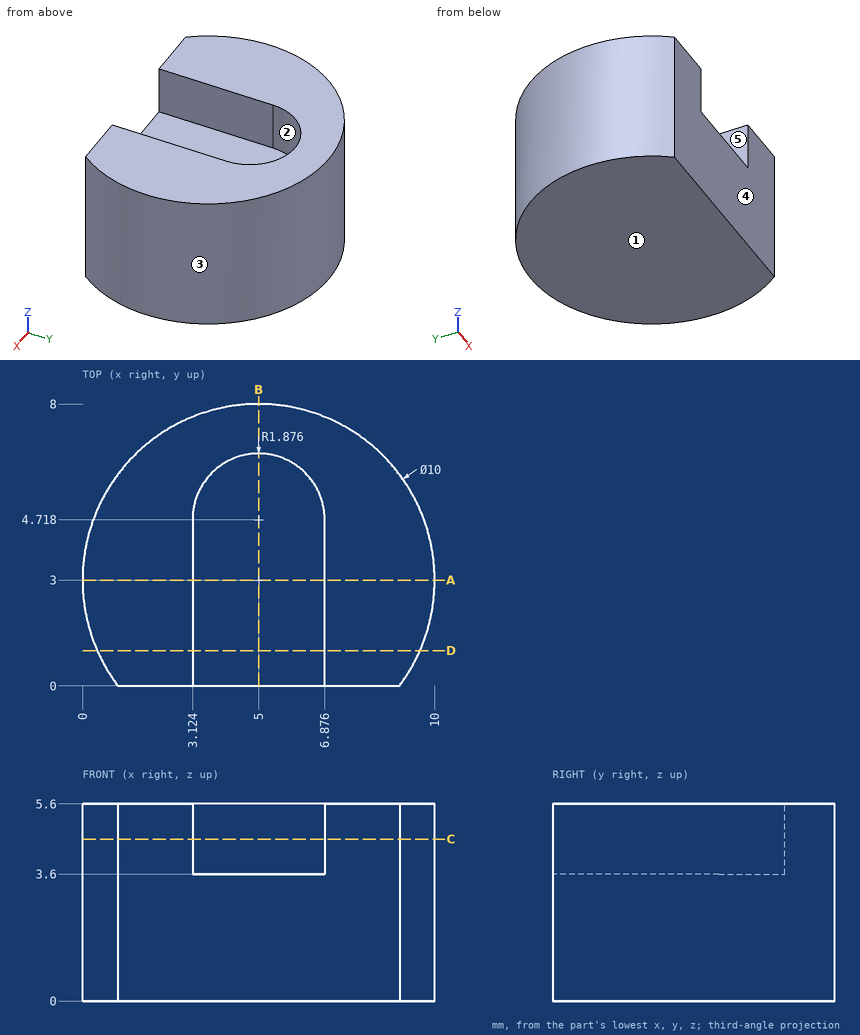
Print and shaded views of the part. All mm, measured from the part's lowest x, y and z. A direction names the side the tool comes from. Give positions to 0.01 mm unless a question says otherwise; leave off trailing zeros. Order: outer loops, then holes, each group sorted by start corner. A loop starts at its lowest first (then second) coordinate and runs counter-clockwise, first axis right, second up. Notation, with made-up numbers: (-26.75, 73) -> (19.25, 73) arc R37 cw to (19.25, 109) -> close; hole circle Ø7 at (50.5, 35.5). An arc over 180 degrees is marked (long way). Use CSV: the item, a comma, the result in double quotes.
1. Band-saw the part on B-B, the plane x = 5. Give the cut face in (y, z).
Outcome:
outline,"(0, 0) -> (8, 0) -> (8, 5.6) -> (6.59, 5.6) -> (6.59, 3.6) -> (0, 3.6) -> close"
2. Mould opens along X. For the marked faces 3, 4 and 5 say: +X half, -X half, draft (parallel to the pull), parting line (faces both ways), or undercut.
Outcome:
face 3,"parting line"
face 4,"draft"
face 5,"undercut"
3. Band-saw the part on D-D, the plane y = 1. Give the cut face in (x, z), then the cut area to 3 significant figures.
Outcome:
outline,"(0.42, 0) -> (9.58, 0) -> (9.58, 5.6) -> (6.88, 5.6) -> (6.88, 3.6) -> (3.12, 3.6) -> (3.12, 5.6) -> (0.42, 5.6) -> close"
area,"43.8 mm²"
4. Band-saw the part on A-A, the plane y = 3. Give the cut face in (x, z).
Outcome:
outline,"(0, 0) -> (10, 0) -> (10, 5.6) -> (6.88, 5.6) -> (6.88, 3.6) -> (3.12, 3.6) -> (3.12, 5.6) -> (0, 5.6) -> close"
5. Drop flat-ended pins along their axis: pin 1 (1 mm diameter, centred on y = 2, z = 4.5, fed in from -X) (1 decimal); pin 2 (0.6 mm diameter, centred on y = 3.5, z = 4, fed in from +X); pin 3 (3 mm diameter, centred on y = 6.5, z = 2.5, fed in from -X). Give the stop position or say it passes through.
Outcome:
pin 1,"x = 0"
pin 2,"x = 10"
pin 3,"x = 0.42"
6. Band-saw the part on C-C, the plane z = 4.6. Give the cut face in (x, y).
Outcome:
outline,"(1, 0) -> (3.12, 0) -> (3.12, 4.72) arc R1.88 cw to (6.88, 4.72) -> (6.88, 0) -> (9, 0) arc R5 ccw (long way) to start"
7. Drill centre lines: line 1 along X through (y, z) = (4.5, 5.35); line 2 along X through (y, z) = (2.25, 4.2); line 3 along Z through (x, y) = (4.5, 2.75). Where is each one in solid material? Low to high. Write a range as from..to.
Outcome:
line 1,"0.23..3.12, 6.88..9.77"
line 2,"0.06..3.12, 6.88..9.94"
line 3,"0..3.6"
8. 3-axis set-ups, long thin cutter, end or side, ignore diameter. For the marked faces 1 and 2: which of +Z, -Z, +X, -X, +Y, -Y reach the whole face in a straight line?
Outcome:
face 1,"-Z, +X, -X, +Y, -Y"
face 2,"+Z, -Y"
